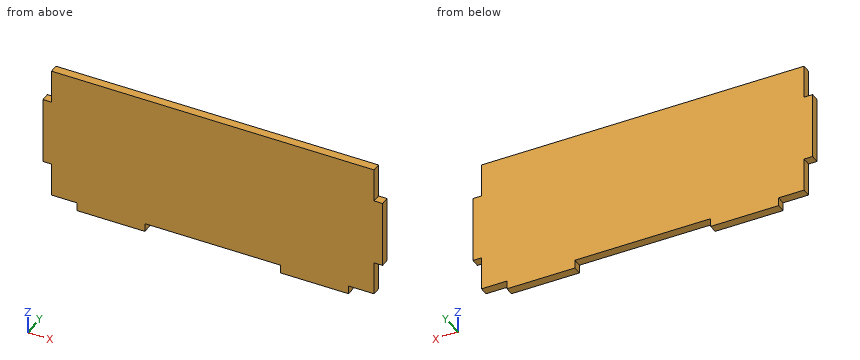
```python
from build123d import *

# Parameters (mm, degrees)
F0_W     = 254
F0_H     = 101.6
F1_DEPTH = 6.35
F2_W     = 50.8
F2_H     = 6.35
F3_DEPTH = 6.35
F4_W     = 6.35
F4_H     = 25.4
F5_DEPTH = 25.4


with BuildPart() as f1:
    # F0 (on Front) → F1 (new body)
    with BuildSketch(Plane.XZ):
        with Locations((0, 50.8)):
            Rectangle(F0_W, F0_H)
    extrude(amount=F1_DEPTH)

    # F2 (on face) → F3 (join)
    with BuildSketch(Plane.XZ.offset(6.35)):
        with Locations((76.2, -3.175)):
            Rectangle(F2_W, F2_H)
        with Locations((-76.2, -3.175)):
            Rectangle(F2_W, F2_H)
    extrude(amount=-F3_DEPTH)

    # F4 (on face) → F5 (cut)
    with BuildSketch(Plane.XZ.offset(6.35)):
        with Locations((123.825, 88.9)):
            Rectangle(F4_W, F4_H)
        with Locations((123.825, 12.7)):
            Rectangle(F4_W, F4_H)
        with Locations((-123.825, 12.7)):
            Rectangle(F4_W, F4_H)
        with Locations((-123.825, 88.9)):
            Rectangle(F4_W, F4_H)
    extrude(amount=-F5_DEPTH, mode=Mode.SUBTRACT)


solid = f1.part
```
Verification items for the finished model (mm, model axes). Coordinates: 2 decimals unless noted, no trailing zeros. Loops run counter-clockwise (first coordinate to the right, second up) from the corner with the lowest first, then second, coordinate; pieces in that order, holes last. Notation, with made-up numbers: (56, 81.5) -> (67, 81.5) arc R34 cw to (67, 111.5) -> close; hole circle Ø10 at (-19, 65.25). An arc over 180 degrees is marked (long way). Answer in a Markdown table with one row per item.
1) Section check A-A (y = -1.25). Record the cut outline in (x, z).
The answers:
| item | result |
|---|---|
| outline | (-127, 25.4) -> (-120.65, 25.4) -> (-120.65, 0) -> (-101.6, 0) -> (-101.6, -6.35) -> (-50.8, -6.35) -> (-50.8, 0) -> (50.8, 0) -> (50.8, -6.35) -> (101.6, -6.35) -> (101.6, 0) -> (120.65, 0) -> (120.65, 25.4) -> (127, 25.4) -> (127, 76.2) -> (120.65, 76.2) -> (120.65, 101.6) -> (-120.65, 101.6) -> (-120.65, 76.2) -> (-127, 76.2) -> close |
2) Section check B-B (z = 13.5). Record the cut outline in (x, y).
The answers:
| item | result |
|---|---|
| outline | (-120.65, -6.35) -> (120.65, -6.35) -> (120.65, 0) -> (-120.65, 0) -> close |
3) Depth check by flat-ended pin: P1, Ø3, axis at x = -113, y = -2, coming from the -Z side; P2, Ø3, axis at y = -4.5, z = -3, coming from the -X side. Enter the tip coordinate at first touch or a pass-through.
The answers:
| item | result |
|---|---|
| P1 | stops at z = 0 |
| P2 | stops at x = -101.6 |
4) Section check C-C (x = 24). Record the cut outline in (y, z), and give its area (3 significant figures).
The answers:
| item | result |
|---|---|
| outline | (-6.35, 0) -> (0, 0) -> (0, 101.6) -> (-6.35, 101.6) -> close |
| area | 645 mm2 |
5) Scan lines: line 1 along X through (y, z) = (-0.75, -1); line 2 along X through (y, z) = (-4.5, 23.5); line 3 along Z through (x, y) = (48, -5.5). Record each from-to range of solid material in increasing order. Write a range as from..to.
The answers:
| item | result |
|---|---|
| line 1 | x = -101.6..-50.8, 50.8..101.6 |
| line 2 | x = -120.65..120.65 |
| line 3 | z = 0..101.6 |
